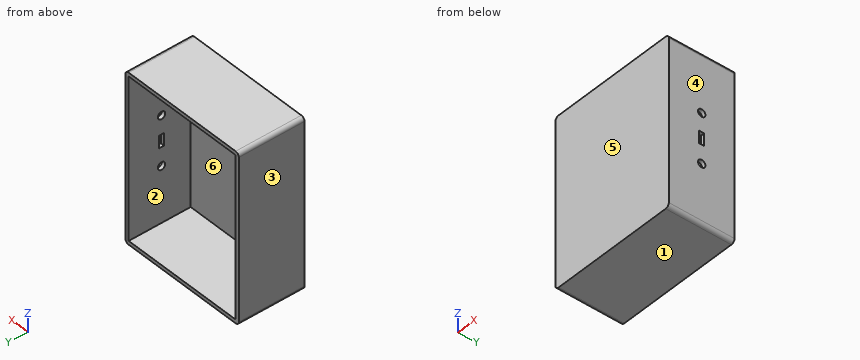
from build123d import *

# Parameters (mm, degrees)
ESQUISSE1_W             = 106
ESQUISSE1_H             = 136
ESQUISSE1_W_2           = 100
ESQUISSE1_H_2           = 130
BOSS_EXTRU_1_DEPTH      = 50
ESQUISSE2_W             = 106
ESQUISSE2_H             = 136
BOSS_EXTRU_2_DEPTH      = 3
CONG_1_R                = 3
ESQUISSE3_R             = 3
ESQUISSE3_W             = 10
ESQUISSE3_H             = 4
ENL_V_MAT_EXTRU_1_DEPTH = 3


with BuildPart() as part:
    # Esquisse1 → Boss.-Extru.1 (new body)
    with BuildSketch(Plane(origin=(0, 0, 0), x_dir=(1, 0, 0), z_dir=(0, 1, 0))):
        Rectangle(ESQUISSE1_W, ESQUISSE1_H)
        Rectangle(ESQUISSE1_W_2, ESQUISSE1_H_2, mode=Mode.SUBTRACT)
    extrude(amount=BOSS_EXTRU_1_DEPTH)

    # Esquisse2 → Boss.-Extru.2 (add)
    with BuildSketch(Plane.XZ):
        Rectangle(ESQUISSE2_W, ESQUISSE2_H)
    extrude(amount=BOSS_EXTRU_2_DEPTH)

    # Congé1
    cong_1_edges = [part.edges().sort_by_distance(p)[0] for p in [
        (53, 23.5, 68),
        (-53, 23.5, 68),
        (-53, 23.5, -68),
        (53, 23.5, -68),
    ]]
    fillet(cong_1_edges, radius=CONG_1_R)

    # Esquisse3 → Enlèv. mat.-Extru.1 (cut)
    with BuildSketch(Plane(origin=(53, 0, 0), x_dir=(0, 0, -1), z_dir=(1, 0, 0))):
        with Locations((-20, 23.5)):
            Circle(ESQUISSE3_R)
        with Locations((20, 23.5)):
            Circle(ESQUISSE3_R)
        with Locations((0, 23.5)):
            Rectangle(ESQUISSE3_W, ESQUISSE3_H)
    extrude(amount=-ENL_V_MAT_EXTRU_1_DEPTH, mode=Mode.SUBTRACT)


solid = part.part
The model under review builds one solid part; all positions refer to its coordinate system, in mm. Face numbers are marked on the shaded views. A direction names the side the tool comes from. Coordinates: 2 decimals unless noted, no trailing zeros. Write each loop counter-clockwise with the first axis right and the second up, starting at its lowest first coordinate (ties: lowest second). Pieces come first, ordered by that corner, then holes. Notation, with made-up numbers: (32, 50) - (86, 50) arc R30 ccw to (86, 88) - close; hole circle Ø9 at (-8.5, 45.5). An arc over 180 degrees is marked (long way). Answer as a JSON object with one key per item and string values. Group by question number.
1. Add section C-C (z = -33.5). Give the boundary of the cut face in (x, y), plus the area to 3 significant figures.
2. Add section D-D (x = 13). Give the boundary of the cut face in (y, z).
3. Machinability: for the marked faces 5 and 6, which of the approach directions +Z, -Z, +X, -X, +Y, -Y give a long, thin tool a straight path to every point of the face, cutting with its end or side? Answer none if there is none.
4. Clearance check with flat-ended pins moving along their axes: pin 1 Ø1 at (x, z) = (29, -51.5) entering from +Y; pin 2 Ø2.5 at (x, y) = (52, 23.5) entering from +Z; pin 3 Ø0.9 at (x, y) = (51.5, 23.5) entering from -Z. State where each tip first meets the part, or that it passes through.
5. Add section A-A (y = 23.5). Give the boundary of the cut face in (x, z).
6. Add section B-B (z = 20). Give the boundary of the cut face in (x, y), plus the area to 3 significant figures.
7. Mouldability with a two-part tool opening along X and no side actions: class the marked faces 1, 2, 3 and 4 as pulls with the +X half, pulls with the -X half, needs draft (parallel to the pull), parting line crosses it, or undercut.
8. To check wall thickness, follow probe 1 along Z at (x, y) = (29, 10.5); probe 2 along X at (y, z) = (24.5, 62); probe 3 along Z at (x, y) = (51, 23). State the ranges of each line that lie inside material, in increasing order.
Findings:
{
 "1": {"outline": "(-53, -3) - (53, -3) - (53, 50) - (50, 50) - (50, 0) - (-50, 0) - (-50, 50) - (-53, 50) - close", "area": "618 mm²"},
 "2": {"outline": "(-3, -68) - (50, -68) - (50, -65) - (0, -65) - (0, 65) - (50, 65) - (50, 68) - (-3, 68) - close"},
 "3": {"face 5": "+Z, -Z, +X, -X, -Y", "face 6": "+Y"},
 "4": {"pin 1": "y = 0", "pin 2": "z = 67.9", "pin 3": "z = -67.81"},
 "5": {"outline": "(-53, -65) arc R3 ccw to (-50, -68) - (50, -68) arc R3 ccw to (53, -65) - (53, -23) - (50, -23) - (50, -65) - (-50, -65) - (-50, 65) - (50, 65) - (50, 23) - (53, 23) - (53, 65) arc R3 ccw to (50, 68) - (-50, 68) arc R3 ccw to (-53, 65) - close; (50, -17) - (53, -17) - (53, -5) - (50, -5) - close; (50, 5) - (53, 5) - (53, 17) - (50, 17) - close"},
 "6": {"outline": "(-53, -3) - (53, -3) - (53, 20.5) - (50, 20.5) - (50, 0) - (-50, 0) - (-50, 50) - (-53, 50) - close; (50, 26.5) - (53, 26.5) - (53, 50) - (50, 50) - close", "area": "600 mm²"},
 "7": {"face 1": "needs draft", "face 2": "undercut", "face 3": "pulls with the -X half", "face 4": "pulls with the +X half"},
 "8": {"probe 1": "-68 to -65, 65 to 68", "probe 2": "-53 to -50, 50 to 53", "probe 3": "-67.83 to -22.96, -17.04 to -5, 5 to 17.04, 22.96 to 67.83"}
}
